Build history of the part. All positions in model axes, mm. Round coordinates to 2 decimals unless told otherwise and drop trailing zeros. Loops run counter-clockwise (first coordinate to the right, second up) from the corner with the lowest first, then second, coordinate; pieces in that order, holes last. Notation, with made-up numbers: M 73,58.25 L 96,58.25 A14 ccw 96,83.25 Z; hole C 27,47 d9. An arc over 180 degrees is marked long. One line per item, written item: value.
```python
from build123d import *

# Parameters (mm, degrees)
F0_W     = 53.34
F0_H     = 7.4762164177
F1_DEPTH = 5.08
F0_W_2   = 15.4877182819
F0_H_2   = 12.8163710635
F0_R     = 1.365180055
F0_R_2   = 1.7356876501
F0_R_3   = 1.2971240832
F2_DEPTH = 5.08
F0_R_4   = 1.201625658
F0_W_3   = 6.0593526471
F0_H_3   = 10.5057700578
F0_W_4   = 49.0457672859
F0_H_4   = 7.3963825689
F0_W_5   = 5.854880067
F0_H_5   = 23.4966807871
F0_R_5   = 1.2613504397
F3_DEPTH = 5.08


with BuildPart() as f1:
    # F0 (on Top) → F1 (new body)
    with BuildSketch(Plane.XY):
        with Locations((102.2345048122, 14.151409833)):
            Rectangle(F0_W, F0_H)
        Polygon((128.9045048122, 10.4133016241), (131.6407098506, 10.4133016241), (134.779159077, 10.4133016241), (134.779159077, 17.8895180418), (128.9045048122, 17.8895180418), align=None)
        Polygon((128.9045048122, -21.6276271147), (128.9045048122, -13.083379163), (75.5645048122, -13.083379163), (75.5645048122, -20.5595947167), (75.5645048122, -22.1616424497), align=None)
        Polygon((75.5645048122, -13.083379163), (75.5645048122, 10.4133016241), (75.5645048122, 17.8895180418), (69.6898505475, 17.8895180418), (69.6898505475, 4.5391316433), (69.6898505475, -8.2772394202), (69.6898505475, -22.1616424497), (75.5645048122, -22.1616424497), (75.5645048122, -20.5595947167), align=None)
    extrude(amount=F1_DEPTH)

    # F0 (on Top) → F2 (join)
    with BuildSketch(Plane.XY):
        with Locations((61.9459914065, -1.8690538884)):
            Rectangle(F0_W_2, F0_H_2)
        with Locations((56.3987791538, -1.916793175)):
            Circle(F0_R, mode=Mode.SUBTRACT)
        with Locations((61.9344774574, -1.8690538884)):
            Circle(F0_R_2, mode=Mode.SUBTRACT)
        with Locations((66.9036880136, -1.6289874911)):
            Circle(F0_R_3, mode=Mode.SUBTRACT)
    extrude(amount=F2_DEPTH)

    # F0 (on Top) → F3 (join)
    with BuildSketch(Plane.XY):
        Polygon((134.779159077, 10.4133016241), (131.6407098506, 10.4133016241), (128.9045048122, 10.4133016241), (128.9045048122, -13.083379163), (131.6407098506, -13.083379163), (134.779159077, -13.083379163), align=None)
        with Locations((133.2313663255, 0)):
            Circle(F0_R_4, mode=Mode.SUBTRACT)
        Polygon((131.6407098506, -13.083379163), (128.9045048122, -13.083379163), (128.9045048122, -21.6276271147), (134.779159077, -21.6276271147), (134.779159077, -13.083379163), align=None)
        with Locations((51.1724559421, -18.3362641919)):
            Rectangle(F0_W_3, F0_H_3)
        with Locations((23.6198959756, -18.3362641919)):
            Rectangle(F0_W_4, F0_H_3)
        Polygon((54.2021322656, -8.2772394202), (54.2021322656, 4.5391316433), (54.2021322656, 10.4133016241), (48.1427796185, 10.4133016241), (48.1427796185, -13.083379163), (54.2021322656, -13.083379163), align=None)
        with Locations((51.1724559421, 14.1114929086)):
            Rectangle(F0_W_3, F0_H_4)
        with Locations((23.6198959756, 14.1114929086)):
            Rectangle(F0_W_4, F0_H_4)
        with Locations((-3.8304277009, 14.1114929086)):
            Rectangle(F0_W_5, F0_H_4)
        with Locations((-3.8304277009, -18.3362641919)):
            Rectangle(F0_W_5, F0_H_3)
        with Locations((-3.8304277009, -1.3350387695)):
            Rectangle(F0_W_5, F0_H_5)
        with Locations((-2.3539937101, 0)):
            Circle(F0_R_5, mode=Mode.SUBTRACT)
    extrude(amount=F3_DEPTH)


solid = f1.part
```
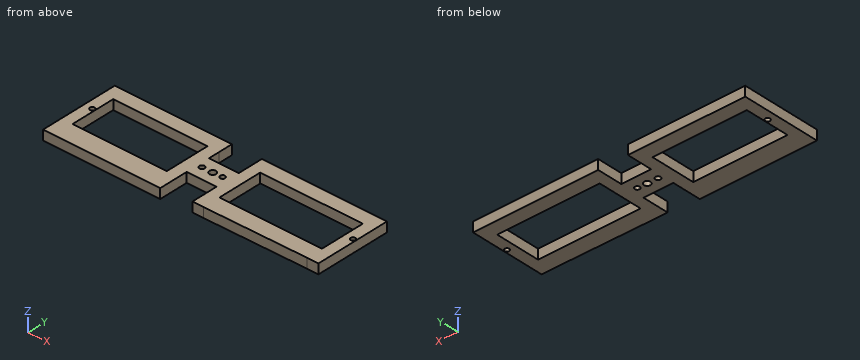
Item 1: Wall check: line 1 along X through (y, z) = (-11, 2.1); line 2 along X through (y, z) = (-4, 3.4); line 3 along X through (y, z) = (11, 0.5). Give the ranges that are in metal, low to high.
Check values:
line 1: x = -6.76 to -0.9, 48.14 to 54.2, 69.69 to 75.56, 128.9 to 134.78
line 2: x = -6.76 to -0.9, 48.14 to 75.56, 128.9 to 134.78
line 3: x = -6.76 to 54.2, 69.69 to 134.78
Item 2: Slice it at C-C, the plane z = 2.65. Give the cut face in (x, y).
Check values:
outline: M -6.76,-23.59 L 54.2,-23.59 L 54.2,-8.28 L 69.69,-8.28 L 69.69,-22.16 L 75.56,-22.16 L 128.9,-21.63 L 134.78,-21.63 L 134.78,17.89 L 69.69,17.89 L 69.69,4.54 L 54.2,4.54 L 54.2,17.81 L -6.76,17.81 Z; hole C -2.35,0 d2.52; hole M -0.9,-13.08 L 48.14,-13.08 L 48.14,10.41 L -0.9,10.41 Z; hole C 56.4,-1.92 d2.73; hole C 61.93,-1.87 d3.47; hole C 66.9,-1.63 d2.59; hole M 75.56,-13.08 L 128.9,-13.08 L 128.9,10.41 L 75.56,10.41 Z; hole C 133.23,0 d2.4
Item 3: Slice it at D-D, the plane y = -18.5. Give the cut face in (x, z), and give its area (3 significant figures).
Check values:
outline: M -6.76,0 L 54.2,0 L 54.2,5.08 L -6.76,5.08 Z; M 69.69,0 L 134.78,0 L 134.78,5.08 L 69.69,5.08 Z
area: 640 mm2
Item 4: Slice it at A-A, the plane x = 19.5. Give the cut face in (y, z), and give its area (3 significant figures).
Check values:
outline: M -23.59,0 L -13.08,0 L -13.08,5.08 L -23.59,5.08 Z; M 10.41,0 L 17.81,0 L 17.81,5.08 L 10.41,5.08 Z
area: 90.9 mm2
Item 5: Slice it at B-B, the plane y = -11. Give the cut face in (x, z), and give its area (3 significant figures).
Check values:
outline: M -6.76,0 L -0.9,0 L -0.9,5.08 L -6.76,5.08 Z; M 48.14,0 L 54.2,0 L 54.2,5.08 L 48.14,5.08 Z; M 69.69,0 L 75.56,0 L 75.56,5.08 L 69.69,5.08 Z; M 128.9,0 L 134.78,0 L 134.78,5.08 L 128.9,5.08 Z
area: 120 mm2
Item 6: Drop flat-ended pins along their axis: P1, Ø2.5, axis at x = 27, z = 2, coming from the +Y side; P2, Ø10, axis at x = 67.5, y = 11.5, coming from the +Z side; P3, Ø2, axis at x = 81.5, z = 2.5, coming from the -Y side; P4, Ø4, axis at x = 37.5, y = 8, coming from the -Z side. Give the stop position or say it passes through.
Check values:
P1: stops at y = 17.81
P2: stops at z = 5.08
P3: stops at y = -22.11
P4: passes through
